from build123d import *

# Parameters (mm, degrees)
F0_W     = 42
F0_H     = 42
F1_DEPTH = 992
F3_DEPTH = 100
F4_R     = 20.99999


# Not quite as in the source:
# - a fillet or chamfer is up to 0.001 mm smaller than in the source, because OpenCascade refuses the exact size


with BuildPart() as f1:
    # F0 (on Front) → F1 (new body)
    with BuildSketch(Plane.XZ):
        Rectangle(F0_W, F0_H)
    extrude(amount=F1_DEPTH)

    # F2 (on face) → F3 (cut)
    with BuildSketch(Plane.YZ.offset(21)):
        Polygon((-950, -21), (-992, 21), (-992, -21), align=None)
    extrude(amount=-F3_DEPTH, mode=Mode.SUBTRACT)

    # F4 (radius 21 in the source; OpenCascade refuses exactly that, so slightly less here)
    f4_edges = [f1.edges().sort_by_distance(p)[0] for p in [
        (-21, -496, 21),
        (-21, -475, -21),
        (21, -496, 21),
        (21, -475, -21),
    ]]
    fillet(f4_edges, radius=F4_R)


solid = f1.part
Can you work these out from the model? Positions are in its coordinate system, mm. Round coordinates to 2 decimals unless told otherwise and drop trailing zeros. Write each loop counter-clockwise with the first axis right and the second up, starting at its lowest first coordinate (ties: lowest second). Pieces come first, ordered by that corner, then holes. Notation, with made-up numbers: M 59,29.5 L 111,29.5 A15 ccw 111,53.5 Z; hole C 62.25,43.5 d11. An arc over 180 degrees is marked long. Use a Markdown table: item, result.
Item 1: If I drill on line 1 along X through (y, z) = (-885, 1.5); line 2 along Z through (x, y) = (-0.5, -791); line 3 along Z through (x, y) = (5, -115), over which ranges is the centre line in solid material (lowest first)? Write a range as [from, to].
Found:
| item | result |
|---|---|
| line 1 | x = [-20.95, 20.95] |
| line 2 | z = [-20.99, 20.99] |
| line 3 | z = [-20.4, 20.4] |
Item 2: For pin 1 Ø8 at (x, y) = (14.5, -320.5) entering from -Z; pin 2 Ø8 at (y, z) = (-676.5, 10) entering from -X; pin 3 Ø1 at (y, z) = (-190.5, 15) entering from -X, each with a flat end and sliding along its axis, tell me the tip position at first contact or that it passes through.
Found:
| item | result |
|---|---|
| pin 1 | stops at z = -18.19 |
| pin 2 | stops at x = -20.12 |
| pin 3 | stops at x = -15.19 |
Item 3: I want a section at B-B (z = 11). List the corners of the cut face in (x, y) for me, and give its area (3 significant figures).
Found:
| item | result |
|---|---|
| outline | M -17.89,-982 L 17.89,-982 L 17.89,0 L -17.89,0 Z |
| area | 35,100 mm2 |
Item 4: I want a section at C-C (x = -14). List the corners of the cut face in (y, z) for me, and give its area (3 significant figures).
Found:
| item | result |
|---|---|
| outline | M -986.65,15.65 L -955.35,-15.65 L 0,-15.65 L 0,15.65 Z |
| area | 30,400 mm2 |
